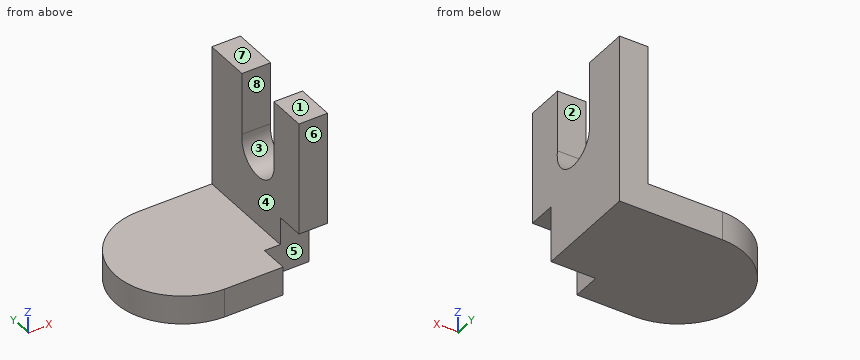
from build123d import *

# Parameters (mm, degrees)
F0_W     = 33.0062359571
F0_H     = 59.3436355703
F1_DEPTH = 12.7
F2_W     = 59.3436355703
F2_H     = 75.1609131694
F3_DEPTH = 12.7
F5_DEPTH = 12.701
F6_W     = 12.7
F6_H     = 12.3074490905
F7_DEPTH = 12.7


with BuildPart() as f1:
    # F0 (on Top) → F1 (new body)
    with BuildSketch(Plane.XY):
        with BuildLine():
            Line((0, -66.963635385), (0, -7.6199998148))
            ThreePointArc((0, -7.6199998148), (-29.1663880378, -37.2918175999), (0, -66.963635385))
        make_face()
        with Locations((16.5031179786, -37.2918175999)):
            Rectangle(F0_W, F0_H)
    extrude(amount=F1_DEPTH)

    # F2 (on face) → F3 (join)
    with BuildSketch(Plane.YZ.offset(33.0062359571)):
        with Locations((-37.2918175999, 37.5804565847)):
            Rectangle(F2_W, F2_H)
    extrude(amount=F3_DEPTH)

    # F4 (on face) → F5 (cut, through all)
    with BuildSketch(Plane(origin=(33.0062359571, 0, 0), x_dir=(0, -1, 0), z_dir=(-1, 0, 0))):
        with BuildLine():
            Line((28.1709097326, 75.1609131694), (28.1709097326, 47.4518202245))
            ThreePointArc((28.1709097326, 47.4518202245), (39.2987808247, 34.7509651719), (49.8763658106, 47.9136370122))
            Line((49.8763658106, 47.9136370122), (49.8763658106, 75.1609131694))
            Line((49.8763658106, 75.1609131694), (28.1709097326, 75.1609131694))
        make_face()
    extrude(amount=-F5_DEPTH, mode=Mode.SUBTRACT)

    # F6 (on face) → F7 (cut)
    with BuildSketch(Plane.XZ.offset(66.963635385)):
        Polygon((33.0062359571, 12.7), (25.9446389973, 12.7), (25.9446389973, 0), (45.7062359571, 0), (45.7062359571, 12.7), align=None)
        with Locations((39.3562359571, 18.8537245452)):
            Rectangle(F6_W, F6_H)
    extrude(amount=-F7_DEPTH, mode=Mode.SUBTRACT)


solid = f1.part
For this review, take the finished solid that the model builds, in its own axes (mm). Face numbers are marked on the shaded views. A direction names the side the tool comes from. Round coordinates to 2 decimals unless told otherwise and drop trailing zeros. Order: outer loops, then holes, each group sorted by start corner. A loop starts at its lowest first (then second) coordinate and runs counter-clockwise, first axis right, second up. Notation, with made-up numbers: (-36.75, 76.5) -> (8.25, 76.5) arc R33 ccw to (8.25, 108.5) -> close; hole circle Ø6 at (21, -3.5). An arc over 180 degrees is marked (long way). Write item = value, one per line. Start each with the question number.
1) Tool access review of the marked faces 4, 5, 6, 7 and 8: name each direction out of +Z, -Z, +X, -X, +Y, -Y from which nothing blocks a thin tool from reaching the whole face with its end or side.
2) Take a section at B-B on y = -59. State the section outline as (x, z) points.
3) Take a section at D-D on x = 12. State the section outline as (y, z) points, plus the area to 3 significant figures.
4) The part is to be moulded in two halves that separate along Z. For the marked faces 1, 2 and 3, say which applies: +Z half, -Z half, draft (parallel to the pull), parting line (faces both ways), or undercut.
5) To check wall thickness, follow line 1 (X direction, y = -63, z = 30); line 2 (Z direction, x = 5, y = -44); line 3 (Y direction, x = 28, z = 8). State the ranges of each line that lie inside material, in increasing order. Write a range as from..to.
6) Insertion check: pin 1 (6 mm diameter, centred on x = 28, y = -23, fed in from +Z); pin 2 (10 mm diameter, centred on x = 37.5, z = 18, fed in from -Y); pin 3 (6.5 mm diameter, centred on y = -61, z = 9, fed in from +X); pin 4 (10 mm diameter, centred on x = 4.5, z = 15.5, fed in from -Y). Each pin has a flat end and moves straight along its axis. Give the tip position at first contact, or say it passes through.
7) Take a section at A-A on z = 69.5. State the section outline as (x, y) points, plus the area to 3 significant figures.
Verdict:
q1.face_4 = +Z, -X, +Y, -Y
q1.face_5 = -Z, +X, -Y
q1.face_6 = +Z, -Z, +X, -X, -Y
q1.face_7 = +Z, +X, -X, +Y, -Y
q1.face_8 = +Z, +X, -X
q2.outline = (-19.72, 0) -> (25.94, 0) -> (25.94, 12.7) -> (-19.72, 12.7) -> close; (33.01, 25.01) -> (45.71, 25.01) -> (45.71, 75.16) -> (33.01, 75.16) -> close
q3.outline = (-66.96, 0) -> (-7.62, 0) -> (-7.62, 12.7) -> (-66.96, 12.7) -> close
q3.area = 754 mm2
q4.face_1 = +Z half
q4.face_2 = draft
q4.face_3 = undercut
q5.line_1 = 33.01..45.71
q5.line_2 = 0..12.7
q5.line_3 = -54.26..-7.62
q6.pin_1 = 12.7
q6.pin_2 = -54.26
q6.pin_3 = 25.94
q6.pin_4 = -66.96
q7.outline = (33.01, -66.96) -> (45.71, -66.96) -> (45.71, -49.88) -> (33.01, -49.88) -> close; (33.01, -28.17) -> (45.71, -28.17) -> (45.71, -7.62) -> (33.01, -7.62) -> close
q7.area = 478 mm2
